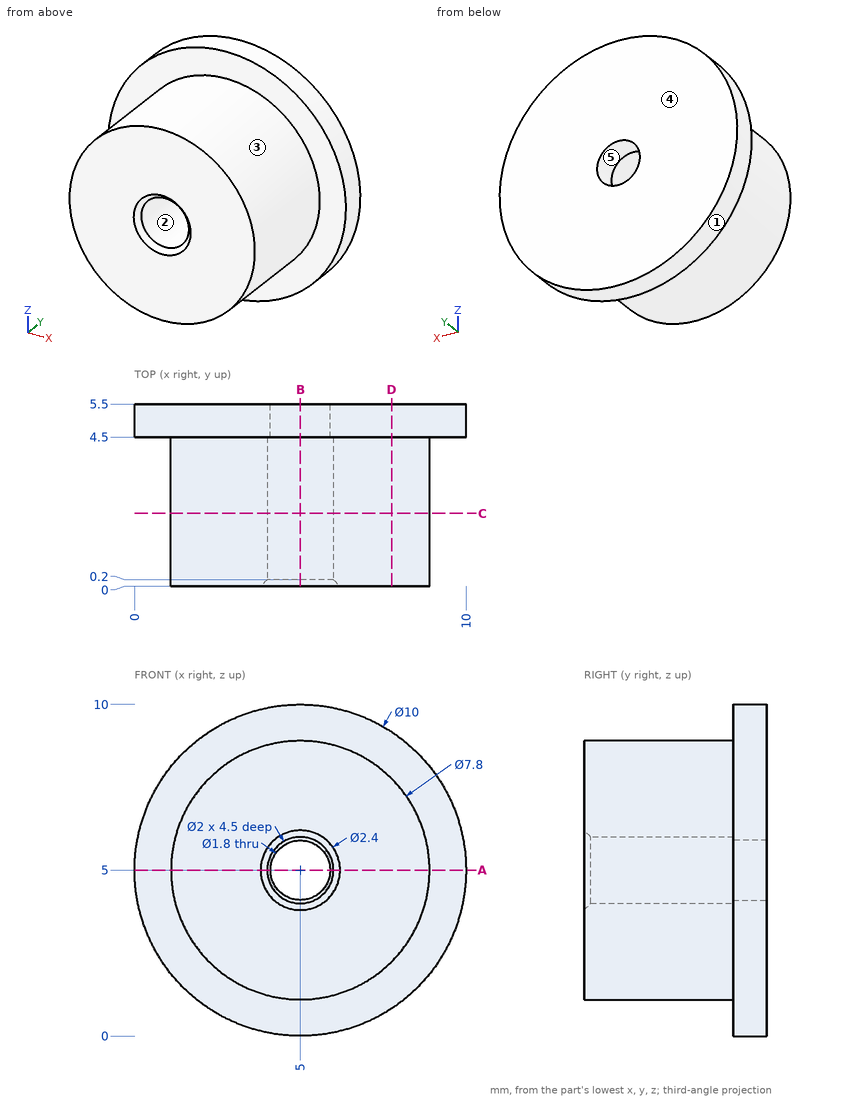
Source: three-view drawing plus pictorial views. Frame: mm from the lowest corner of the part. A direction names the side the tool comes from. Round coordinates to 2 decimals unless told otherwise and drop trailing zeros. Loops run counter-clockwise (first coordinate to the right, second up) from the corner with the lowest first, then second, coordinate; pieces in that order, holes last.
Q1. Mould query, pull axis X, two halves, no side actions, for the marked faces 3, 4 and 5. Classes: pulls with the +X half, pulls with the -X half, needs draft (parallel to the pull), parting line crosses it, or undercut.
Q2. Section D-D, the plane x = 7.75. Return loops of the section in (y, z).
Q3. Access query for the marked faces 1 and 2. Directions: +Z, -Z, +X, -X, +Y, -Y. A direction counts if a zero-diameter tool reaches every point of the face in a straight line with its end or side. Return the directions, or none.
Q4. Ray query, line 1 (X direction, y = 4.9, z = 5); line 2 (X direction, y = 1.5, z = 5); line 3 (Y direction, x = 1, z = 3.25). Return the intervals inside material, ascending.
Q5. Section B-B, the plane x = 5. Return loops of the section in (y, z), plus the area to 3 significant figures.
Q6. Section A-A, the plane z = 5. Return loops of the section in (x, y).
Q7. Section C-C, the plane y = 2.2. Return loops of the section in (x, z), plus the area to 3 significant figures.
Q8. First-contact query: P1, Ø1, axis at x = 4, y = 1, coming from the +Z side; P2, Ø3, axis at x = 9, y = 1.5, coming from the -Z side. Flat tips, straight axial feed; report the tip coordinate or a pass-through.
Solutions:
1. face 3: parting line crosses it
1. face 4: needs draft
1. face 5: undercut
2. outline: (0, 2.23) - (4.5, 2.23) - (4.5, 0.82) - (5.5, 0.82) - (5.5, 9.18) - (4.5, 9.18) - (4.5, 7.77) - (0, 7.77) - close
3. face 1: +Y, -Y
3. face 2: -Y
4. line 1: x = 0 to 4.1, 5.9 to 10
4. line 2: x = 1.1 to 4, 6 to 8.9
4. line 3: y = 4.5 to 5.5
5. outline: (0, 1.1) - (4.5, 1.1) - (4.5, 0) - (5.5, 0) - (5.5, 4.1) - (4.5, 4.1) - (4.5, 4) - (0.2, 4) - (0, 3.8) - close; (0, 6.2) - (0.2, 6) - (4.5, 6) - (4.5, 5.9) - (5.5, 5.9) - (5.5, 10) - (4.5, 10) - (4.5, 8.9) - (0, 8.9) - close
5. area: 34.3 mm2
6. outline: (0, 4.5) - (1.1, 4.5) - (1.1, 0) - (3.8, 0) - (4, 0.2) - (4, 4.5) - (4.1, 4.5) - (4.1, 5.5) - (0, 5.5) - close; (5.9, 4.5) - (6, 4.5) - (6, 0.2) - (6.2, 0) - (8.9, 0) - (8.9, 4.5) - (10, 4.5) - (10, 5.5) - (5.9, 5.5) - close
7. outline: circle Ø7.8 at (5, 5); hole circle Ø2 at (5, 5)
7. area: 44.6 mm2
8. P1: stops at z = 8.87
8. P2: stops at z = 2.01
